Could you check a few things on this model? Use its own coordinates, in mm. A direction names the side the tool comes from. Give positions to 0.01 mm unless a question says otherwise; leave off trailing zeros. Loops run counter-clockwise (first coordinate to the right, second up) from the corner with the lowest first, then second, coordinate; pieces in that order, holes last. Notation, with made-up numbers: (41.25, -11) -> (51.25, -11) arc R32 cw to (51.25, 20) -> close; hole circle Ø8 at (14, 81.5). An arc over 180 degrees is marked (long way). Put each result on its own line as item: value.
```python
from build123d import *

# Parameters (mm, degrees)
F1_DEPTH = 12
F2_R     = 5.25
F3_DEPTH = 2


with BuildPart() as f1:
    # F0 (on Right) → F1 (new body)
    with BuildSketch(Plane.YZ):
        with BuildLine():
            Line((6, 0), (-6, 0))
            add(Edge.make_bspline(
                [(-15.0137397329, -11.5619591722), (-13.5906271424, -11.2964920093), (-10.7601897079, -9.2903086336), (-6.4181021832, -4.7073575718), (-6.1370336878, -1.4182246783), (-6, 0)],
                knots=[0, 0, 0, 0, 0.3207224524, 0.6871017532, 1, 1, 1, 1], degree=3))
            Line((-15.0137397329, -11.5619591722), (-25.0122166845, -11.7364832366))
            Line((-25.0122166845, -11.7364832366), (-25, -12.4363766232))
            Line((-25, -12.4363766232), (54.9878156125, -11.0401841082))
            Line((54.9878156125, -11.0401841082), (54.9748430875, -8.0402121561))
            add(Edge.make_bspline(
                [(6, 0), (6.3458147236, -1.1588554342), (7.4985462399, -5.0603049881), (30.6654186689, -7.0675654114), (46.5840497498, -8.0880688799), (54.9748430875, -8.0402121561)],
                knots=[0, 0, 0, 0, 0.1686157391, 0.5621249017, 1, 1, 1, 1], degree=3))
        make_face()
    extrude(amount=F1_DEPTH)

    # F2 (on face) → F3 (cut)
    with BuildSketch(Plane.XY):
        with Locations((6, 0)):
            Circle(F2_R)
    extrude(amount=-F3_DEPTH, mode=Mode.SUBTRACT)


solid = f1.part
```
1. Thinking about a two-plate mould opening in X: for faces 1 (the face through (2.13, 3.55, -0.99)), 2 (the face through (5.9, 5.4, 0)), 3 (the face through (12, 14, -8)), which applies, pulls with the +X half, pulls with the -X half, needs draft (parallel to the pull), parting line crosses it, or undercut?
Recorded:
face 1: undercut
face 2: needs draft
face 3: pulls with the +X half
2. If we section it at A-A (y = 0): List the corners of the cut face in (x, z) for me.
Recorded:
outline: (0, -12) -> (12, -12) -> (12, 0) -> (11.25, 0) -> (11.25, -2) -> (0.75, -2) -> (0.75, 0) -> (0, 0) -> close
3. For faces 4 (the face through (6, 0, -2)), 5 (the face through (0, 14, -8)), which set-ups out of +Z, -Z, +X, -X, +Y, -Y let a thin tool reach every point of the face, with its end or its side?
Recorded:
face 4: +Z
face 5: +Z, -Z, -X, +Y, -Y
4. I'm going to push flat-ended pins straight in: pin 1 (1.5 mm diameter, centred on x = 2, z = -5.5, fed in from -Y); pin 2 (3 mm diameter, centred on x = 6, y = -2, fed in from +Z); pin 3 (2 mm diameter, centred on x = 1.5, y = -5, fed in from -Z); pin 4 (6 mm diameter, centred on y = 38, z = -2.5, fed in from +X). Where does each tip first touch, or does it pass through?
Recorded:
pin 1: stops at y = -8.11
pin 2: stops at z = -2
pin 3: stops at z = -12.1
pin 4: passes through
5. I need wall thicknesses on line 1 (X direction, y = -1, z = -1); line 2 (Y direction, x = 6, z = -1.4); line 3 (Y direction, x = 6, z = -0.6). Which ranges of each line are inside material? Lowest first, please.
Recorded:
line 1: x = 0 to 0.85, 11.15 to 12
line 2: y = -6.15 to -5.25, 5.25 to 6.49
line 3: y = -6.06 to -5.25, 5.25 to 6.18
